```python
from build123d import *

# Parameters (mm, degrees)
SKETCH_1_W          = 15
SKETCH_1_H          = 15
SKETCH_1_W_2        = 13
SKETCH_1_H_2        = 13
EXTRUDE_1_DEPTH     = 250
SKETCH_3_R          = 2
CUT_EXTRUDE_2_DEPTH = 251.561868607
SKETCH_5_R          = 2.5
SKETCH_5_R_2        = 2
CUT_EXTRUDE_4_DEPTH = 251.561868607


with BuildPart() as part:
    # 草图1 → 凸台-拉伸1 (new body)
    with BuildSketch(Plane(origin=(0, 0, 0), x_dir=(1, 0, 0), z_dir=(0, 1, 0))):
        Rectangle(SKETCH_1_W, SKETCH_1_H)
        Rectangle(SKETCH_1_W_2, SKETCH_1_H_2, mode=Mode.SUBTRACT)
    extrude(amount=EXTRUDE_1_DEPTH)

    # 草图3 → 切除-拉伸2 (cut, through all)
    with BuildSketch(Plane.XY.offset(7.5)):
        with Locations((0, 240)):
            Circle(SKETCH_3_R)
        with Locations((0, 220)):
            Circle(SKETCH_3_R)
        with Locations(Location((0, 30, 0), (0, 0, 180))):
            Circle(SKETCH_3_R)
        with Locations(Location((0, 10, 0), (0, 0, 180))):
            Circle(SKETCH_3_R)
        with Locations((0, 200)):
            Circle(SKETCH_3_R)
        with Locations(Location((0, 50, 0), (0, 0, 180))):
            Circle(SKETCH_3_R)
    extrude(amount=-CUT_EXTRUDE_2_DEPTH, mode=Mode.SUBTRACT)

    # 草图5 → 切除-拉伸4 (cut, through all)
    with BuildSketch(Plane(origin=(7.5, 0, 0), x_dir=(0, 0, -1), z_dir=(1, 0, 0))):
        with Locations((0, 140)):
            Circle(SKETCH_5_R)
        with Locations((0, 110)):
            Circle(SKETCH_5_R)
        with Locations((0, 170)):
            Circle(SKETCH_5_R_2)
        with Locations((0, 80)):
            Circle(SKETCH_5_R_2)
    extrude(amount=-CUT_EXTRUDE_4_DEPTH, mode=Mode.SUBTRACT)


solid = part.part
```
Geometry check sheet. Reference: the model listing, model coordinates, mm. A direction names the side the tool comes from. Coordinates: 2 decimals unless noted, no trailing zeros. Write each loop counter-clockwise with the first axis right and the second up, starting at its lowest first coordinate (ties: lowest second). Pieces come first, ordered by that corner, then holes. Notation, with made-up numbers: M 2.5,6 L 35.5,6 A10 ccw 35.5,12 Z; hole C 45,58 d9. An arc over 180 degrees is marked long. Answer as a JSON object with one key per item and string values.
1. Section check A-A, the plane y = 140. Enter the section's corners in (x, z).
Answers below:
{"outline": "M -7.5,-7.5 L 7.5,-7.5 L 7.5,-2.5 L 6.5,-2.5 L 6.5,-6.5 L -6.5,-6.5 L -6.5,-2.5 L -7.5,-2.5 Z; M -7.5,2.5 L -6.5,2.5 L -6.5,6.5 L 6.5,6.5 L 6.5,2.5 L 7.5,2.5 L 7.5,7.5 L -7.5,7.5 Z"}
2. Tool access check on faces 1 (the flat face through (-6.5, 123, 0)), 2 (the flat face through (-7, 250, 0)). Record the directions out of +Z, -Z, +X, -X, +Y, -Y that give a thin tool (end or side, any length) a straight path to the whole face; none if there is none.
Answers below:
{"face 1": "+Y, -Y", "face 2": "+Z, -Z, +X, -X, +Y"}
3. Draft check along X on faces 3 (the cylindrical face through (0, 8, 7)), 4 (the cylindrical face through (-6.99, 112.48, 0.33)). Enter one of: released by +X, released by -X, zero draft, split by the parting line, or undercut.
Answers below:
{"face 3": "undercut", "face 4": "zero draft"}
4. Scan lines: L1, parallel to Z at x = 0.5, y = 143.5; L2, parallel to X at y = 10, z = -7.25. Record each from-to range of solid material in increasing order.
Answers below:
{"L1": "z = -7.5 to -6.5, 6.5 to 7.5", "L2": "x = -7.5 to -2, 2 to 7.5"}
5. Section check B-B, the plane y = 68. Enter the section's corners in (x, z).
Answers below:
{"outline": "M -7.5,-7.5 L 7.5,-7.5 L 7.5,7.5 L -7.5,7.5 Z; hole M -6.5,-6.5 L 6.5,-6.5 L 6.5,6.5 L -6.5,6.5 Z"}
